```python
from build123d import *

# Parameters (mm, degrees)
POCKET_DEPTH       = 432.177804
POLARPATTERN_COUNT = 4
POLARPATTERN_ANGLE = 180
SKETCH006_W        = 30
SKETCH006_H        = 75
POCKET001_DEPTH    = 72


with BuildPart() as part:
    # Sketch → Revolution001 (revolve)
    with BuildSketch(Plane.XZ):
        Polygon((47.75, 29.8), (55.5, 29.8), (55.5, 105.8), (59.5, 105.8), (59.5, 25.8), (47.75, 25.8), align=None)
    revolve(axis=Axis((0, 0, 0), (0, 0, 1)))

    # Sketch005 → Pocket (cut, through all)
    with BuildSketch(Plane.YZ):
        Polygon((0, 35.8), (-17.5, 65.8), (0, 95.8), (17.5, 65.8), align=None)
    pocket = extrude(amount=-POCKET_DEPTH, mode=Mode.SUBTRACT)

    # PolarPattern: Pocket ×4 about axis
    polarpattern_axis = Axis((0, 0, 0), (0, 0, 1))
    for i in range(1, POLARPATTERN_COUNT):
        add(pocket.rotate(polarpattern_axis, i * POLARPATTERN_ANGLE / (POLARPATTERN_COUNT - 1)), mode=Mode.SUBTRACT)

    # Sketch006 (on Face7 of PolarPattern) → Pocket001 (cut)
    with BuildSketch(Plane(origin=(0, 0, 105.8), x_dir=(-1, 0, 0), z_dir=(0, 0, 1))):
        with Locations((0, -37.5)):
            Rectangle(SKETCH006_W, SKETCH006_H)
    extrude(amount=-POCKET001_DEPTH, mode=Mode.SUBTRACT)


solid = part.part
```
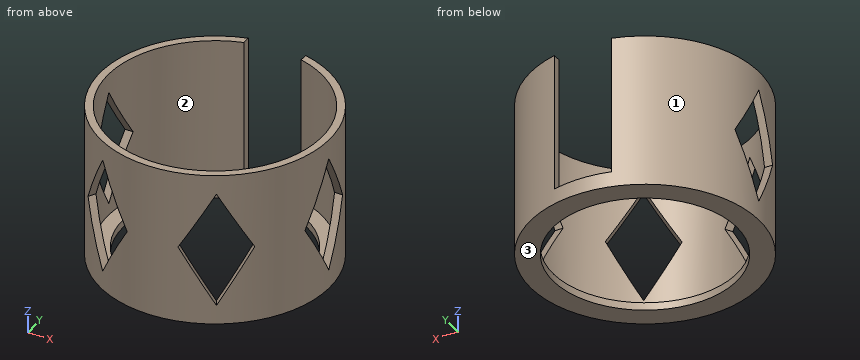
For this review, take the finished solid that the model builds, in its own axes (mm). Face numbers are marked on the shaded views. Round coordinates to 2 decimals unless told otherwise and drop trailing zeros. Write each loop counter-clockwise with the first axis right and the second up, starting at its lowest first coordinate (ties: lowest second). Pieces come first, ordered by that corner, then holes. Notation, with made-up numbers: (43, 59.5) - (61, 59.5) arc R19 cw to (61, 75.5) - close; hole circle Ø7 at (48, 21). An arc over 180 degrees is marked (long way). Answer as CSV lines item,"result". Start each with the question number.
(1) For pin 1 (3.5 mm diameter, centred on y = 55, z = 85.5, fed in from +X); pin 2 (1 mm diameter, centred on x = -47.5, z = 97.5, fed in from -Y); pin 3 (1.5 mm diameter, centred on y = -18.5, z = 97.5, fed in from +X); pin 4 (1 mm diameter, centred on y = -47.5, z = 80.5, fed in from +X), all flat-tipped, find the tip position at first contact; note any pin that passes through.
(2) Add section D-D, the plane y = -6.5. State the section outline as (x, z) points, plus the area to 3 significant figures.
(3) Add section B-B, the plane y = 46. State the section outline as (x, z) points.
(4) For line 1 (Y direction, x = 0, z = 29); line 2 (Z direction, x = -36.5, y = -32.5); line 3 (Y direction, x = 0, z = 66.5), list the stretches that pass through material, from the lowest coordinate up.
(5) Add section C-C, the plane z = 71.5. State the section outline as (x, y) points (3 decimals).
(6) Mouldability with a two-part tool opening along X and no side actions: class the marked faces 1, 2 and 3 as +X half, -X half, draft (parallel to the pull), parting line (faces both ways), or undercut.
(7) Add section A-A, the plane x = 0. State the section outline as (y, z) points, plus the area to 3 significant figures.
From the geometry:
1,pin 1,"stops at x = 26.55"
1,pin 2,"stops at y = -36.49"
1,pin 3,"stops at x = 56.79"
1,pin 4,"passes through"
2,outline,"(-59.14, 25.8) - (-47.31, 25.8) - (-47.31, 29.8) - (-55.12, 29.8) - (-55.12, 46.94) - (-59.14, 46.94) - close; (-59.14, 84.66) - (-55.12, 84.66) - (-55.12, 105.8) - (-59.14, 105.8) - close; (47.31, 25.8) - (59.14, 25.8) - (59.14, 46.94) - (55.12, 46.94) - (55.12, 29.8) - (47.31, 29.8) - close; (55.12, 84.66) - (59.14, 84.66) - (59.14, 105.8) - (55.12, 105.8) - close"
2,area,"403 mm²"
3,outline,"(-37.74, 25.8) - (-12.81, 25.8) - (-12.81, 29.8) - (-31.05, 29.8) - (-31.05, 105.8) - (-37.74, 105.8) - close; (12.81, 25.8) - (37.74, 25.8) - (37.74, 105.8) - (31.05, 105.8) - (31.05, 29.8) - (12.81, 29.8) - close"
4,line 1,"y = -59.5 to -47.75, 47.75 to 59.5"
4,line 2,"z = 25.8 to 29.8"
4,line 3,"y = -59.5 to -55.5"
5,outline,"(-57.787, -14.175) arc R59.5 ccw to (-41.169, -42.957) - (-39.106, -39.383) arc R55.5 cw to (-53.659, -14.175) - close; (-57.787, 14.175) - (-53.659, 14.175) arc R55.5 cw to (-15, 53.435) - (-15, 57.578) arc R59.5 ccw to start; (-16.618, -57.132) arc R59.5 ccw to (16.618, -57.132) - (14.554, -53.558) arc R55.5 cw to (-14.554, -53.558) - close; (15, 53.435) arc R55.5 cw to (53.659, 14.175) - (57.787, 14.175) arc R59.5 ccw to (15, 57.578) - close; (39.106, -39.383) - (41.169, -42.957) arc R59.5 ccw to (57.787, -14.175) - (53.659, -14.175) arc R55.5 cw to start"
6,face 1,"parting line"
6,face 2,"undercut"
6,face 3,"draft"
7,outline,"(-59.5, 25.8) - (-47.75, 25.8) - (-47.75, 29.8) - (-55.5, 29.8) - (-55.5, 105.8) - (-59.5, 105.8) - close; (47.75, 25.8) - (59.5, 25.8) - (59.5, 33.8) - (55.5, 33.8) - (55.5, 29.8) - (47.75, 29.8) - close"
7,area,"414 mm²"
